For this review, use the dimensioned drawing (mm, ordinates from the lowest corner) and the shaded views. A direction names the side the tool comes from. Give positions to 0.01 mm unless a question says otherwise; leave off trailing zeros. Loops run counter-clockwise (first coordinate to the right, second up) from the corner with the lowest first, then second, coordinate; pieces in that order, holes last. Notation, with made-up numbers: M 77.25,41 L 82.25,41 A24 cw 82.25,65 Z; hole C -14,9.5 d9. An arc over 180 degrees is marked long. Use a Markdown table: item, result. Add a question column.
(1) For the marked faces 1, 2 and 3, list the 3-axis set-ups (+Z, -Z, +X, -X, +Y, -Y) from which the entire face can be reached by the end or side of a thin tool; tool diameter is ignored.
(2) Add section C-C, the plane z = 56. Give the boundary of the cut face in (x, y), then the cut area to 3 significant figures.
(3) Add section D-D, the plane x = 21. Give the boundary of the cut face in (y, z).
(4) Insertion check: pin 1 Ø2.5 at (x, z) = (14, 56) entering from -Y; pin 2 Ø3 at (x, z) = (7.5, 28.5) entering from -Y; pin 3 Ø0.5 at (y, z) = (1, 56.5) entering from -X. Each pin has a flat end and moves straight along its axis. Give the tip position at first contact, or say it passes through.
(5) Add section B-B, the plane y = 1.2. Give the boundary of the cut face in (x, z), then the cut area to 3 significant figures.
(6) For probe 1 along X at (y, z) = (0.95, 54.5); probe 2 along Y at (x, z) = (15.25, 52.5); probe 3 along Z at (x, y) = (23.5, 0.7), list the stretches that pass through material, from the lowest coordinate up.
(7) Add section A-A, the plane x = 9. Give the boundary of the cut face in (y, z), then the cut area to 3 significant figures.
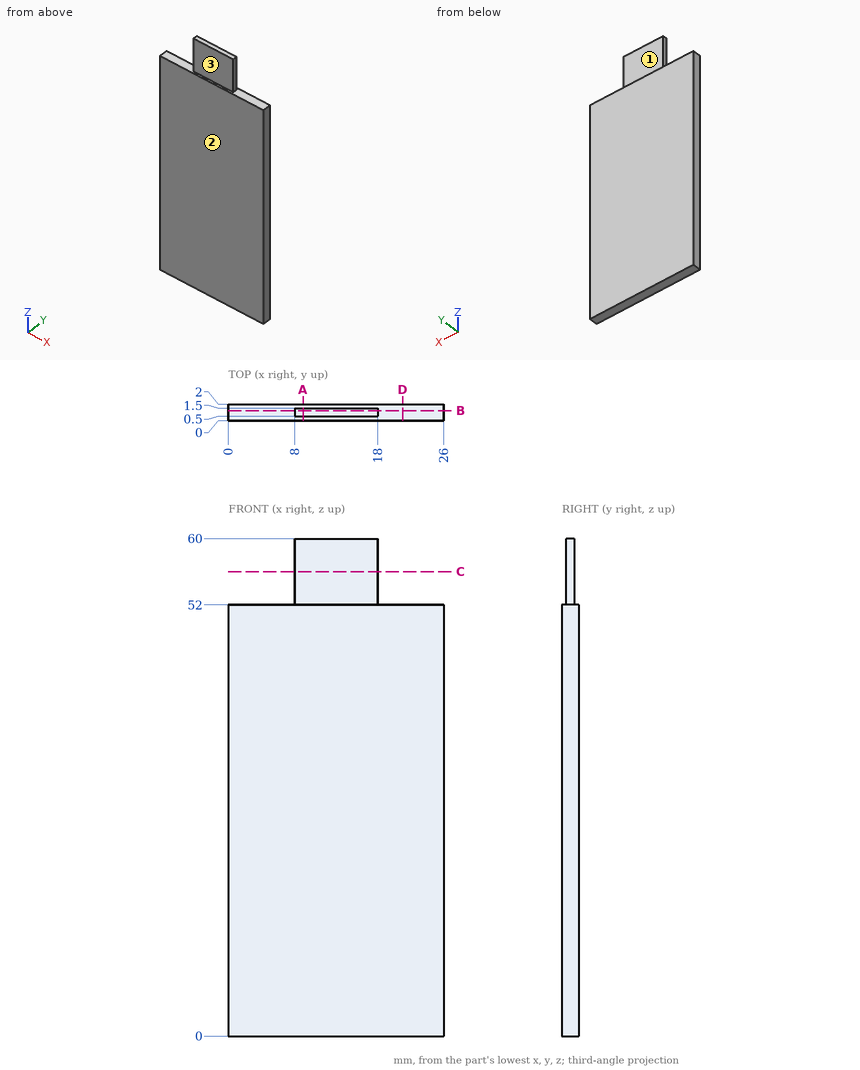
Established:
| question | item | result |
|---|---|---|
| 1 | face 1 | +Z, +X, -X, +Y |
| 1 | face 2 | +Z, -Z, +X, -X, -Y |
| 1 | face 3 | +Z, +X, -X, -Y |
| 2 | outline | M 8,0.5 L 18,0.5 L 18,1.5 L 8,1.5 Z |
| 2 | area | 10.0 mm^2 |
| 3 | outline | M 0,0 L 2,0 L 2,52 L 0,52 Z |
| 4 | pin 1 | y = 0.5 |
| 4 | pin 2 | y = 0 |
| 4 | pin 3 | x = 8 |
| 5 | outline | M 0,0 L 26,0 L 26,52 L 18,52 L 18,60 L 8,60 L 8,52 L 0,52 Z |
| 5 | area | 1,430 mm^2 |
| 6 | probe 1 | 8 to 18 |
| 6 | probe 2 | 0.5 to 1.5 |
| 6 | probe 3 | 0 to 52 |
| 7 | outline | M 0,0 L 2,0 L 2,52 L 1.5,52 L 1.5,60 L 0.5,60 L 0.5,52 L 0,52 Z |
| 7 | area | 112 mm^2 |
